from build123d import *

# Parameters (mm, degrees)
F1_DEPTH = 3
F2_DEPTH = 10


with BuildPart() as f1:
    # F0 (on Top) → F1 (new body)
    with BuildSketch(Plane.XY):
        with BuildLine():
            Line((28.379236, 17.204217), (-33.620764, 17.204217))
            Line((-33.620764, 17.204217), (-33.620764, 11.454217))
            Line((-33.620764, 11.454217), (37.929236, 11.454217))
            Line((37.929236, 11.454217), (37.929236, 29.454217))
            Line((37.929236, 29.454217), (-33.620764, 29.454217))
            Line((-33.620764, 29.454217), (-33.620764, 23.704217))
            Line((-33.620764, 23.704217), (28.379236, 23.704217))
            ThreePointArc((28.379236, 23.704217), (31.629236, 20.454217), (28.379236, 17.204217))
        make_face()
    extrude(amount=F1_DEPTH)

    # F0 (on Top) → F2 (join)
    with BuildSketch(Plane.XY):
        with BuildLine():
            Line((-33.620764, 18.954217), (-33.620764, 17.204217))
            Line((-33.620764, 17.204217), (28.379236, 17.204217))
            ThreePointArc((28.379236, 17.204217), (31.629236, 20.454217), (28.379236, 23.704217))
            Line((28.379236, 23.704217), (-33.620764, 23.704217))
            Line((-33.620764, 23.704217), (-33.620764, 21.954217))
            Line((-33.620764, 21.954217), (28.379236, 21.954217))
            ThreePointArc((28.379236, 21.954217), (29.879236, 20.454217), (28.379236, 18.954217))
            Line((28.379236, 18.954217), (-33.620764, 18.954217))
        make_face()
        with BuildLine():
            ThreePointArc((-33.620764, 23.704217), (-36.870764, 20.454217), (-33.620764, 17.204217))
            Line((-33.620764, 17.204217), (-33.620764, 18.954217))
            ThreePointArc((-33.620764, 18.954217), (-35.120764, 20.454217), (-33.620764, 21.954217))
            Line((-33.620764, 21.954217), (-33.620764, 23.704217))
        make_face()
    extrude(amount=F2_DEPTH)


solid = f1.part
The model under review builds one solid part; all positions refer to its coordinate system, in mm. A direction names the side the tool comes from. Round coordinates to 2 decimals unless told otherwise and drop trailing zeros. Order: outer loops, then holes, each group sorted by start corner. A loop starts at its lowest first (then second) coordinate and runs counter-clockwise, first axis right, second up. Notation, with made-up numbers: (33.5, 2.25) -> (43.5, 2.25) arc R17 ccw to (43.5, 22.25) -> close; hole circle Ø1 at (80, 86.5). An arc over 180 degrees is marked (long way). Return JSON: item names as keys, results as strings.
1. Take a section at C-C (y = 13.5). Write out the cut boundary in (x, z), then the cut area to 3 significant figures.
Answer block:
{"outline": "(-33.62, 0) -> (37.93, 0) -> (37.93, 3) -> (-33.62, 3) -> close", "area": "215 mm²"}
2. For faces 4 (the face through (-3, 17.204, 6)), 5 (the face through (-3, 21.954, 5)), 6 (the face through (-33.621, 14, 1)), list the 3-axis set-ups (+Z, -Z, +X, -X, +Y, -Y) from which the entire face can be reached by the end or side of a thin tool; tool diameter is ignored.
Answer block:
{"face 4": "+Z, +X, -X, -Y", "face 5": "+Z, -Z", "face 6": "+Z, -Z, -X, -Y"}
3. The part is to be moulded in two halves that separate along Y. For faces 1 (the face through (-2, 23.704, 6)), 2 (the face through (29.88, 20.49, 4.93)), 3 (the face through (2, 17, 3)), say which applies: +Y half, -Y half, draft (parallel to the pull), parting line (faces both ways), or undercut.
Answer block:
{"face 1": "+Y half", "face 2": "undercut", "face 3": "draft"}
4. Insertion check: P1, Ø3, axis at x = -23, y = 15, coming from the -Z side; P2, Ø2.5, axis at y = 14, z = 1.5, coming from the -X side; P3, Ø3.5, axis at x = -17.5, z = 7.5, coming from the -Y side; P4, Ø3, axis at y = 17.5, z = 3, coming from the -X side. Each pin has a flat end and moves straight along its axis. Give the tip position at first contact, or say it passes through.
Answer block:
{"P1": "stops at z = 0", "P2": "stops at x = -33.62", "P3": "stops at y = 17.2", "P4": "stops at x = -36.53"}
5. For L1, parallel to Y at x = 18.5, z = 2.5; L2, parallel to Y at x = 16, z = 5.75; L3, parallel to X at y = 20.25, z = 8.5, list the stretches that pass through material, from the lowest coordinate up. Write a range as [from, to].
Answer block:
{"L1": "y = [11.45, 18.95], [21.95, 29.45]", "L2": "y = [17.2, 18.95], [21.95, 23.7]", "L3": "x = [-36.86, -35.11], [29.87, 31.62]"}
6. Take a section at A-A (x = 20). Write out the cut boundary in (y, z), then the cut area to 3 significant figures.
Answer block:
{"outline": "(11.45, 0) -> (18.95, 0) -> (18.95, 10) -> (17.2, 10) -> (17.2, 3) -> (11.45, 3) -> close; (21.95, 0) -> (29.45, 0) -> (29.45, 3) -> (23.7, 3) -> (23.7, 10) -> (21.95, 10) -> close", "area": "69.5 mm²"}
7. Take a section at B-B (z = 2.25). Write out the cut boundary in (x, y).
Answer block:
{"outline": "(-33.62, 11.45) -> (37.93, 11.45) -> (37.93, 29.45) -> (-33.62, 29.45) -> (-33.62, 23.7) arc R3.25 ccw to (-33.62, 17.2) -> close; hole (-33.62, 18.95) -> (28.38, 18.95) arc R1.5 ccw to (28.38, 21.95) -> (-33.62, 21.95) arc R1.5 ccw to start"}
